The model under review builds one solid part; all positions refer to its coordinate system, in mm. A direction names the side the tool comes from. Give positions to 0.01 mm unless a question says otherwise; leave off trailing zeros. Order: outer loops, then holes, each group sorted by start corner. A loop starts at its lowest first (then second) coordinate and runs counter-clockwise, first axis right, second up.
```python
from build123d import *

# Parameters (mm, degrees)
SKETCH1_W               = 150
SKETCH1_H               = 70
BOSS_EXTRUDE1_DEPTH     = 15
SKETCH2_W               = 15
SKETCH2_H               = 70
BOSS_EXTRUDE2_DEPTH     = 120
CUT_EXTRUDE1_DEPTH      = 151
SKETCH5_R               = 10
CUT_EXTRUDE2_DEPTH      = 125
CUT_EXTRUDE2_DEPTH_BACK = 5
FILLET1_R               = 4
SKETCH6_R               = 15
CUT_EXTRUDE3_DEPTH      = 5


with BuildPart() as part:
    # Sketch1 → Boss-Extrude1 (new body)
    with BuildSketch(Plane(origin=(0, 0, 0), x_dir=(0, 0, -1), z_dir=(1, 0, 0))):
        Rectangle(SKETCH1_W, SKETCH1_H)
    extrude(amount=BOSS_EXTRUDE1_DEPTH)

    # Sketch2 → Boss-Extrude2 (add)
    with BuildSketch(Plane(origin=(15, 0, 0), x_dir=(0, 0, -1), z_dir=(1, 0, 0))):
        with Locations((-67.5, 0)):
            Rectangle(SKETCH2_W, SKETCH2_H)
        with Locations((67.5, 0)):
            Rectangle(SKETCH2_W, SKETCH2_H)
    extrude(amount=BOSS_EXTRUDE2_DEPTH)

    # Sketch3 → Cut-Extrude1 (cut, through all)
    with BuildSketch(Plane.XY.offset(75)):
        with BuildLine():
            ThreePointArc((99.999999969, 35), (124.748737331, 24.748737352), (135, 0))
            Line((135, 0), (135, 35))
            Line((135, 35), (99.999999969, 35))
        make_face()
        with BuildLine():
            Line((100, -35), (135, -35))
            Line((135, -35), (135, 0))
            ThreePointArc((135, 0), (124.748737342, -24.748737342), (100, -35))
        make_face()
    extrude(amount=-CUT_EXTRUDE1_DEPTH, mode=Mode.SUBTRACT)

    # Sketch5 → Cut-Extrude2 (cut, two sides)
    with BuildSketch(Plane(origin=(0, 0, 60), x_dir=(-1, 0, 0), z_dir=(0, 0, -1))) as cut_extrude2_sk:
        with Locations((-100, 0)):
            Circle(SKETCH5_R)
    extrude(amount=CUT_EXTRUDE2_DEPTH, mode=Mode.SUBTRACT)
    extrude(cut_extrude2_sk.sketch, amount=-CUT_EXTRUDE2_DEPTH_BACK, mode=Mode.SUBTRACT)

    # Fillet1
    fillet1_edges = [part.edges().sort_by_distance(p)[0] for p in [
        (49.999999985, 35, 75),
        (49.999999985, 35, -75),
        (135, 1.5e-08, 75),
        (135, 1.5e-08, -75),
        (0, 0, 75),
        (50, -35, -75),
        (50, -35, 75),
        (0, 0, -75),
    ]]
    fillet(fillet1_edges, radius=FILLET1_R)

    # Sketch6 → Cut-Extrude3 (cut)
    with BuildSketch(Plane.ZY):
        Circle(SKETCH6_R)
    extrude(amount=-CUT_EXTRUDE3_DEPTH, mode=Mode.SUBTRACT)


solid = part.part
```
Item 1: For faces 1 (the flat face through (15, 0, 1)), 2 (the cylindrical face through (2.465, 0.66, -14.985)), 3 (the flat face through (13, -35, 0)), 4 (the flat face through (100, 0, -65)), list the 3-axis set-ups (+Z, -Z, +X, -X, +Y, -Y) from which the entire face can be reached by the end or side of a thin tool; tool diameter is ignored.
Values found:
face 1: +X, +Y, -Y
face 2: -X
face 3: +Z, -Z, +X, -X, -Y
face 4: none
Item 2: Take a section at B-B (z = 0). Give the boundary of the cut face in (x, y), and give its area (3 significant figures).
Values found:
outline: (0, -35) - (15, -35) - (15, 35) - (0, 35) - (0, 15) - (5, 15) - (5, -15) - (0, -15) - close
area: 900 mm2
Item 3: Take a section at A-A (x = 79). Give the boundary of the cut face in (y, z), and give its area (3 significant figures).
Values found:
outline: (-35, -71) arc R4 ccw to (-31, -75) - (31, -75) arc R4 ccw to (35, -71) - (35, -60) - (-35, -60) - close; (-35, 60) - (35, 60) - (35, 71) arc R4 ccw to (31, 75) - (-31, 75) arc R4 ccw to (-35, 71) - close
area: 2,090 mm2
Item 4: For line 1 (Y direction, x = 100, z = 63.1); line 2 (Z direction, x = 44.5, y = 24); line 3 (X direction, y = 0, z = -62), list the stretches that pass through material, from the lowest coordinate up.
Values found:
line 1: y = -35 to -10, 10 to 35
line 2: z = -75 to -60, 60 to 75
line 3: x = 0 to 90, 110 to 135
Item 5: Take a section at C-C (z = 29). Give the boundary of the cut face in (x, y).
Values found:
outline: (0, -35) - (15, -35) - (15, 35) - (0, 35) - close
Item 6: Draft analysis for pull direction X (two halves, no side actions). For faces 5 (the flat face through (5, 0, 0)), 6 (the cylindrical face through (110, 0, 62)), 7 (the flat face through (100, 0, 65)), 8 (the flat face through (67, 0, -75)), state which applies: released by +X, released by -X, zero draft, split by the parting line, or undercut.
Values found:
face 5: released by -X
face 6: undercut
face 7: undercut
face 8: zero draft
Item 7: Clearance check with flat-ended pins moving along their axes: pin 1 Ø24 at (y, z) = (7, 7) entering from -X; pin 2 Ø1 at (y, z) = (-10, -50) entering from +X. State where each tip first meets the part, or that it passes through.
Values found:
pin 1: stops at x = 0
pin 2: stops at x = 15
